Source: three-view drawing plus pictorial views. Frame: mm from the lowest corner of the part. A direction names the side the tool comes from. Coordinates: 2 decimals unless noted, no trailing zeros. Loops run counter-clockwise (first coordinate to the right, second up) from the corner with the lowest first, then second, coordinate; pieces in that order, holes last. Notation, with made-up numbers: (66.5, 71.25) - (83.5, 71.25) arc R12 cw to (83.5, 79.25) - close; hole circle Ø1 at (-32, 76.5). An arc over 180 degrees is marked (long way). Return JSON: item names as keys, results as strings.
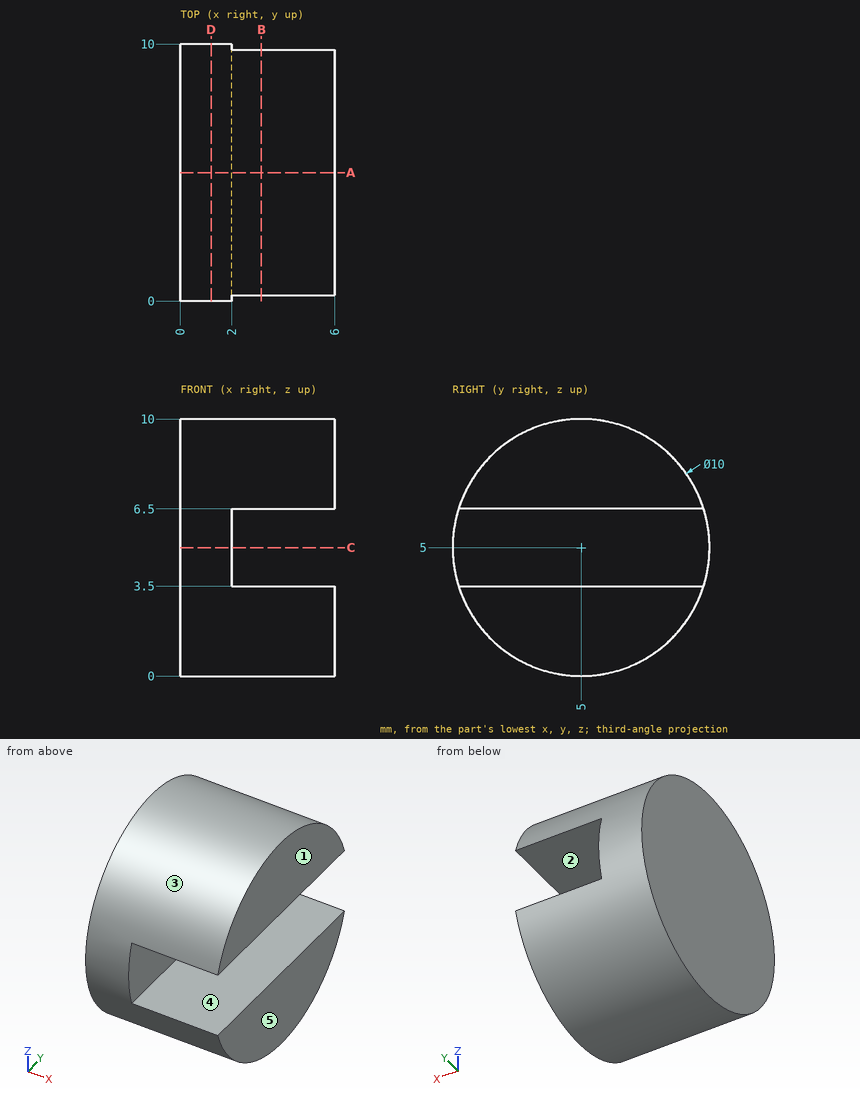
Item 1: Mould query, pull axis Z, two halves, no side actions, for the marked faces 3, 4 and 5. Classes: +Z half, -Z half, draft (parallel to the pull), parting line (faces both ways), or undercut.
Worked out:
{"face 3": "parting line", "face 4": "undercut", "face 5": "draft"}
Item 2: First-contact query: pin 1 Ø0.9 at (y, z) = (6.5, 5) entering from +X; pin 2 Ø1.2 at (x, y) = (4.5, 6) entering from -Z; pin 3 Ø2 at (x, y) = (4.5, 2.5) entering from +Z. Flat tips, straight axial feed; report the tip coordinate or a pass-through.
Worked out:
{"pin 1": "x = 2", "pin 2": "z = 0.02", "pin 3": "z = 9.77"}
Item 3: Section query C-C, the plane z = 5. Return loops of the section in (x, y).
Worked out:
{"outline": "(0, 0) - (2, 0) - (2, 10) - (0, 10) - close"}
Item 4: Ray query, probe 1 along Z at (x, y) = (2.95, 6.5); probe 2 along X at (y, z) = (7.75, 4); probe 3 along Z at (x, y) = (5.25, 9). Return the intervals inside material, ascending. Write a range as from..to.
Worked out:
{"probe 1": "0.23..3.5, 6.5..9.77", "probe 2": "0..2", "probe 3": "2..3.5, 6.5..8"}
Item 5: Reachability of the marked faces 1 and 2 from +Z, -Z, +X, -X, +Y, -Y: full face, straight path, thin tool, end or side. Return the list, or none.
Worked out:
{"face 1": "+Z, -Z, +X, +Y, -Y", "face 2": "+X, +Y, -Y"}
Item 6: Section query D-D, the plane x = 1.2. Return loops of the section in (y, z).
Worked out:
{"outline": "circle Ø10 at (5, 5)"}
Item 7: Section query A-A, the plane y = 5. Return loops of the section in (x, z), and give its area (3 significant figures).
Worked out:
{"outline": "(0, 0) - (6, 0) - (6, 3.5) - (2, 3.5) - (2, 6.5) - (6, 6.5) - (6, 10) - (0, 10) - close", "area": "48.0 mm^2"}
Item 8: Section query B-B, the plane x = 3.15. Return loops of the section in (y, z).
Worked out:
{"outline": "(0.23, 3.5) arc R5 ccw to (9.77, 3.5) - close; (0.23, 6.5) - (9.77, 6.5) arc R5 ccw to start"}
